Geometry: final body of the model. Coordinates: model frame, mm. A direction names the side the tool comes from. Give positions to 0.01 mm unless a question says otherwise; leave off trailing zeros. Loops run counter-clockwise (first coordinate to the right, second up) from the corner with the lowest first, then second, coordinate; pieces in that order, holes last. Notation, with made-up numbers: (29, 19.5) -> (74, 19.5) arc R23 ccw to (74, 47.5) -> close; hole circle Ø3 at (76.5, -29). An arc over 180 degrees is marked (long way). Answer in a Markdown table with one row per item. Add a question column.
from build123d import *

# Parameters (mm, degrees)
SKIZZE1_R                       = 2.35
AUFSATZ_LINEAR_AUSTRAGEN1_DEPTH = 30
SKIZZE4_R                       = 1.55
SCHNITT_LINEAR_AUSTRAGEN2_DEPTH = 6
SKIZZE5_R                       = 10
AUFSATZ_LINEAR_AUSTRAGEN3_DEPTH = 5
SCHNITT_LINEAR_START            = -5
SKIZZE6_R                       = 12.190209649
SCHNITT_LINEAR_AUSTRAGEN3_DEPTH = 5


with BuildPart() as part:
    # Skizze1 → Aufsatz-Linear austragen1 (new body)
    with BuildSketch(Plane.XY):
        Circle(SKIZZE1_R)
    extrude(amount=AUFSATZ_LINEAR_AUSTRAGEN1_DEPTH)

    # Skizze4 → Schnitt-Linear austragen2 (cut)
    with BuildSketch(Plane(origin=(0, 0, 0), x_dir=(-1, 0, 0), z_dir=(0, 0, -1))):
        Circle(SKIZZE4_R)
    extrude(amount=-SCHNITT_LINEAR_AUSTRAGEN2_DEPTH, mode=Mode.SUBTRACT)

    # Skizze5 → Aufsatz-Linear austragen3 (add)
    with BuildSketch(Plane.XY.offset(30)):
        Circle(SKIZZE5_R)
    extrude(amount=AUFSATZ_LINEAR_AUSTRAGEN3_DEPTH)

    # Skizze6 → Schnitt-Linear austragen3 (cut)
    with BuildSketch(Plane.XY.offset(35).offset(SCHNITT_LINEAR_START)):
        Circle(SKIZZE6_R)
        with BuildLine():
            ThreePointArc((0, 10), (0.840722593, 9.609503215), (1.736481777, 9.84807753))
            ThreePointArc((1.736481777, 9.84807753), (2.49662285, 9.317523323), (3.420201433, 9.396926208))
            ThreePointArc((3.420201433, 9.396926208), (4.076664484, 8.742435199), (5, 8.660254038))
            ThreePointArc((5, 8.660254038), (5.532838731, 7.901712605), (6.427876097, 7.660444431))
            ThreePointArc((6.427876097, 7.660444431), (6.820900473, 6.820900473), (7.660444431, 6.427876097))
            ThreePointArc((7.660444431, 6.427876097), (7.901712605, 5.532838731), (8.660254038, 5))
            ThreePointArc((8.660254038, 5), (8.742435199, 4.076664484), (9.396926208, 3.420201433))
            ThreePointArc((9.396926208, 3.420201433), (9.317523323, 2.49662285), (9.84807753, 1.736481777))
            ThreePointArc((9.84807753, 1.736481777), (9.609503215, 0.840722593), (10, 0))
            ThreePointArc((10, 0), (9.609503215, -0.840722593), (9.84807753, -1.736481777))
            ThreePointArc((9.84807753, -1.736481777), (9.317523323, -2.49662285), (9.396926208, -3.420201433))
            ThreePointArc((9.396926208, -3.420201433), (8.742435199, -4.076664484), (8.660254038, -5))
            ThreePointArc((8.660254038, -5), (7.901712605, -5.532838731), (7.660444431, -6.427876097))
            ThreePointArc((7.660444431, -6.427876097), (6.820900473, -6.820900473), (6.427876097, -7.660444431))
            ThreePointArc((6.427876097, -7.660444431), (5.532838731, -7.901712605), (5, -8.660254038))
            ThreePointArc((5, -8.660254038), (4.076664484, -8.742435199), (3.420201433, -9.396926208))
            ThreePointArc((3.420201433, -9.396926208), (2.49662285, -9.317523323), (1.736481777, -9.84807753))
            ThreePointArc((1.736481777, -9.84807753), (0.840722593, -9.609503215), (0, -10))
            ThreePointArc((0, -10), (-0.840722593, -9.609503215), (-1.736481777, -9.84807753))
            ThreePointArc((-1.736481777, -9.84807753), (-2.49662285, -9.317523323), (-3.420201433, -9.396926208))
            ThreePointArc((-3.420201433, -9.396926208), (-4.076664484, -8.742435199), (-5, -8.660254038))
            ThreePointArc((-5, -8.660254038), (-5.532838731, -7.901712605), (-6.427876097, -7.660444431))
            ThreePointArc((-6.427876097, -7.660444431), (-6.820900473, -6.820900473), (-7.660444431, -6.427876097))
            ThreePointArc((-7.660444431, -6.427876097), (-7.901712605, -5.532838731), (-8.660254038, -5))
            ThreePointArc((-8.660254038, -5), (-8.742435199, -4.076664484), (-9.396926208, -3.420201433))
            ThreePointArc((-9.396926208, -3.420201433), (-9.317523323, -2.49662285), (-9.84807753, -1.736481777))
            ThreePointArc((-9.84807753, -1.736481777), (-9.609503215, -0.840722593), (-10, 0))
            ThreePointArc((-10, 0), (-9.609503215, 0.840722593), (-9.84807753, 1.736481777))
            ThreePointArc((-9.84807753, 1.736481777), (-9.317523323, 2.49662285), (-9.396926208, 3.420201433))
            ThreePointArc((-9.396926208, 3.420201433), (-8.742435199, 4.076664484), (-8.660254038, 5))
            ThreePointArc((-8.660254038, 5), (-7.901712605, 5.532838731), (-7.660444431, 6.427876097))
            ThreePointArc((-7.660444431, 6.427876097), (-6.820900473, 6.820900473), (-6.427876097, 7.660444431))
            ThreePointArc((-6.427876097, 7.660444431), (-5.532838731, 7.901712605), (-5, 8.660254038))
            ThreePointArc((-5, 8.660254038), (-4.076664484, 8.742435199), (-3.420201433, 9.396926208))
            ThreePointArc((-3.420201433, 9.396926208), (-2.49662285, 9.317523323), (-1.736481777, 9.84807753))
            ThreePointArc((-1.736481777, 9.84807753), (-0.840722593, 9.609503215), (0, 10))
        make_face(mode=Mode.SUBTRACT)
    extrude(amount=SCHNITT_LINEAR_AUSTRAGEN3_DEPTH, mode=Mode.SUBTRACT)


solid = part.part
(1) Cut plane B-B on y = 1. Return the cut outline in (x, z), then the cut area to 3 significant figures.
(2) Material intervals for line 1 along Y through (x, z) = (0, 2.4); line 2 along Z through (x, y) = (-2.5, 3); line 3 along X through (y, z) = (-4.5, 33), sorted ascending. Write a range as from..to.
(3) Cut plane D-D on z = 9.5. Return the cut outline in (x, y), then the cut area to 3 significant figures.
(4) Pin query (flat end, axial travel): pin 1 Ø12 at (y, z) = (3.5, 31) entering from -X; pin 2 Ø8 at (y, z) = (4.5, 13) entering from -X; pin 3 Ø5 at (x, z) = (-5.5, 8.5) entering from -Y; pin 4 Ø4 at (x, z) = (-2, 6) entering from -Y. Return the tip coordinate at first contact, or that it passes through.
(5) Draft query along X for faces 1 (the cylindrical face through (-6.81, -6.83, 32.47)), 2 (the cylindrical face through (9.321, -2.484, 32.465)), 3 (the cylindrical face through (-0.83, -9.61, 32.47)). Return one class per face: +X half, -X half, draft (parallel to the pull), parting line (faces both ways), or undercut.
(6) Cut plane A-A on z = 2. Return the cut outline in (x, y).
(7) Reachability of faces 4 (the cylindrical face through (4.089, -8.737, 32.465)), 5 (the flat face through (0, 0, 6)) from +Z, -Z, +X, -X, +Y, -Y: full face, straight path, thin tool, end or side. Return the list, or none.
Answer list:
| question | item | result |
|---|---|---|
| 1 | outline | (-9.6, 30) -> (-2.13, 30) -> (-2.13, 0) -> (-1.18, 0) -> (-1.18, 6) -> (1.18, 6) -> (1.18, 0) -> (2.13, 0) -> (2.13, 30) -> (9.6, 30) -> (9.6, 35) -> (-9.6, 35) -> close |
| 1 | area | 209 mm² |
| 2 | line 1 | y = -2.35..-1.55, 1.55..2.35 |
| 2 | line 2 | z = 30..35 |
| 2 | line 3 | x = -8.62..8.62 |
| 3 | outline | circle Ø4.7 at (0, 0) |
| 3 | area | 17.3 mm² |
| 4 | pin 1 | stops at x = -10 |
| 4 | pin 2 | stops at x = -2.3 |
| 4 | pin 3 | passes through |
| 4 | pin 4 | stops at y = -2.35 |
| 5 | face 1 | -X half |
| 5 | face 2 | +X half |
| 5 | face 3 | undercut |
| 6 | outline | circle Ø4.7 at (0, 0); hole circle Ø3.1 at (0, 0) |
| 7 | face 4 | +Z, -Z, -Y |
| 7 | face 5 | -Z |
